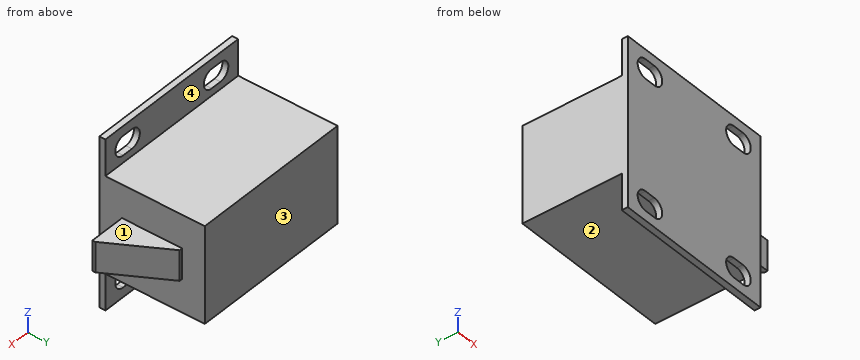
from build123d import *

# Parameters (mm, degrees)
SKETCH083_W   = 27
SKETCH083_H   = 16
PAD049_DEPTH  = 17.5
SKETCH084_W   = 5
SKETCH084_H   = 10
PAD050_DEPTH  = 6
CHAMFER_SIZE2 = 9.5
CHAMFER_SIZE  = 5.5
SKETCH085_W   = 27
SKETCH085_H   = 6
PAD051_DEPTH  = 1


with BuildPart() as part:
    # Sketch083 → Pad049 (new body)
    with BuildSketch(Plane.XZ):
        Rectangle(SKETCH083_W, SKETCH083_H)
    extrude(amount=-PAD049_DEPTH)

    # Sketch084 (on Face4 of Pad049) → Pad050 (join)
    with BuildSketch(Plane(origin=(13.5, 0, 0), x_dir=(0, 0, 1), z_dir=(1, 0, 0))):
        with Locations((0, -8.75)):
            Rectangle(SKETCH084_W, SKETCH084_H)
    extrude(amount=PAD050_DEPTH)

    # Chamfer
    chamfer_edges = [part.edges().sort_by_distance(p)[0] for p in [
        (19.5, 13.75, 0),
    ]]
    chamfer_side = part.faces().sort_by_distance((16.5, 13.75, 0))[0]
    chamfer(chamfer_edges, length=CHAMFER_SIZE, length2=CHAMFER_SIZE2, reference=chamfer_side)

    # Sketch085 (on Face9 of Chamfer) → Pad051 (join)
    with BuildSketch(Plane.XZ):
        with Locations((0, 11)):
            Rectangle(SKETCH085_W, SKETCH085_H)
        with BuildLine():
            Line((-9.9, 9.2), (-8.1, 9.2))
            ThreePointArc((-8.1, 9.2), (-6.5, 10.8), (-8.1, 12.4))
            Line((-8.1, 12.4), (-9.9, 12.4))
            ThreePointArc((-9.9, 12.4), (-11.5, 10.8), (-9.9, 9.2))
        make_face(mode=Mode.SUBTRACT)
        with BuildLine():
            Line((8.1, 9.2), (9.9, 9.2))
            ThreePointArc((9.9, 9.2), (11.5, 10.8), (9.9, 12.4))
            Line((9.9, 12.4), (8.1, 12.4))
            ThreePointArc((8.1, 12.4), (6.5, 10.8), (8.1, 9.2))
        make_face(mode=Mode.SUBTRACT)
        with Locations((0, -11)):
            Rectangle(SKETCH085_W, SKETCH085_H)
        with BuildLine():
            Line((-9.9, -12.4), (-8.1, -12.4))
            ThreePointArc((-8.1, -12.4), (-6.5, -10.8), (-8.1, -9.2))
            Line((-8.1, -9.2), (-9.9, -9.2))
            ThreePointArc((-9.9, -9.2), (-11.5, -10.8), (-9.9, -12.4))
        make_face(mode=Mode.SUBTRACT)
        with BuildLine():
            Line((8.1, -12.4), (9.9, -12.4))
            ThreePointArc((9.9, -12.4), (11.5, -10.8), (9.9, -9.2))
            Line((9.9, -9.2), (8.1, -9.2))
            ThreePointArc((8.1, -9.2), (6.5, -10.8), (8.1, -12.4))
        make_face(mode=Mode.SUBTRACT)
    extrude(amount=-PAD051_DEPTH)


with BuildPart() as part_1:
    # Body020 placement: moved
    add(part.part.moved(Location((16, -46, -47.5))))


solid = part_1.part
Verification items for the finished model (mm, model axes). Face numbers are marked on the shaded views. A direction names the side the tool comes from. Coordinates: 2 decimals unless noted, no trailing zeros. Order: outer loops, then holes, each group sorted by start corner. A loop starts at its lowest first (then second) coordinate and runs counter-clockwise, first axis right, second up. Notation, with made-up numbers: M 64,-20 L 78,-20 A25 ccw 78,4 Z; hole C 89.5,55 d8. An arc over 180 degrees is marked long. One line per item, written item: value. Start each with the question number.
Item 1: Sectioned sample at C-C on x = 9. Record the cut outline in (y, z), then the cut area to 3 significant figures.
Item 2: Depth check by flat-ended pin: P1, Ø6, axis at x = 22, y = -31, coming from the +Z side; P2, Ø3, axis at x = 10.5, z = -35, coming from the +Y side; P3, Ø1, axis at x = 16.5, y = -39, coming from the -Z side. Enter the tip coordinate at first touch or a pass-through.
Item 3: Access from +Z, -Z, +X, -X, +Y, -Y to the whole of each face (thin tool, end or side, straight path). Record for the marked faces 1, 2, 3 and 4.
Item 4: Sectioned sample at A-A on x = 14. Record the cut outline in (y, z), then the cut area to 3 significant figures.
Item 5: Sectioned sample at D-D on y = -38.25. Record the cut outline in (x, z), then the cut area to 3 significant figures.
Item 6: Sectioned sample at B-B on z = -36.7. Record the cut outline in (x, y), then the cut area to 3 significant figures.
Item 7: Thickness scan on probe 1 along X at (y, z) = (-39.5, -40.5); probe 2 along Z at (x, y) = (10, -38); probe 3 along Y at (x, z) = (12, -35.5). Record the ranges inside material, lowest first.
Calculated:
1. outline: M -46,-61.5 L -45,-61.5 L -45,-59.46 L -46,-59.46 Z; M -46,-57.14 L -45,-57.14 L -45,-55.5 L -28.5,-55.5 L -28.5,-39.5 L -45,-39.5 L -45,-37.86 L -46,-37.86 Z; M -46,-35.54 L -45,-35.54 L -45,-33.5 L -46,-33.5 Z
1. area: 287 mm^2
2. P1: z = -39.5
2. P2: y = -45
2. P3: z = -55.5
3. face 1: +Z, +X, +Y, -Y
3. face 2: -Z, +X, -X, +Y
3. face 3: +Z, -Z, +X, -X, +Y
3. face 4: +Z, +X, -X, +Y
4. outline: M -46,-61.5 L -45,-61.5 L -45,-55.5 L -28.5,-55.5 L -28.5,-39.5 L -45,-39.5 L -45,-33.5 L -46,-33.5 Z
4. area: 292 mm^2
5. outline: M 2.5,-55.5 L 29.5,-55.5 L 29.5,-50 L 33.47,-50 L 33.47,-45 L 29.5,-45 L 29.5,-39.5 L 2.5,-39.5 Z
5. area: 452 mm^2
6. outline: M 2.5,-46 L 4.5,-46 L 4.5,-45 L 2.5,-45 Z; M 9.5,-46 L 22.5,-46 L 22.5,-45 L 9.5,-45 Z; M 27.5,-46 L 29.5,-46 L 29.5,-45 L 27.5,-45 Z
6. area: 17.0 mm^2
7. probe 1: 2.5 to 29.5
7. probe 2: -55.5 to -39.5
7. probe 3: -46 to -45
